Model file for the job. Use its own axes, mm. Face numbers are marked on the shaded views. A direction names the side the tool comes from. Round coordinates to 2 decimals unless told otherwise and drop trailing zeros. Write each loop counter-clockwise with the first axis right and the second up, starting at its lowest first coordinate (ties: lowest second). Pieces come first, ordered by that corner, then holes. Notation, with made-up numbers: (-36.5, -36) - (-23.5, -36) arc R24 ccw to (-23.5, -26) - close; hole circle Ø8 at (11.25, 43.25). An arc over 180 degrees is marked (long way). One line per item, written item: value.
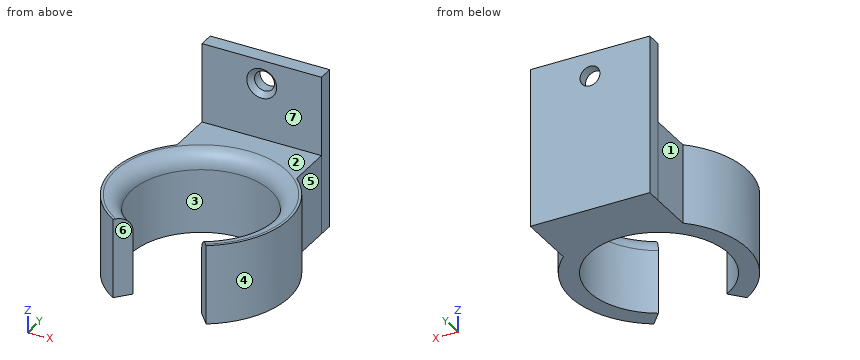
from build123d import *

# Parameters (mm, degrees)
F1_DEPTH       = 25.4
F0_W           = 38.142491
F0_H           = 4.7625
F2_DEPTH       = 50.8
F4_D           = 6.35
F4_CSINK_D     = 9.525
F4_CSINK_ANGLE = 90
F5_R           = 5.08


with BuildPart() as f1:
    # F0 (on Top) → F1 (new body)
    with BuildSketch(Plane.XY):
        with BuildLine():
            Line((-26.27681, 54.485713), (-64.419301, 54.485713))
            Line((-64.419301, 54.485713), (-64.419301, 49.723213))
            Line((-64.419301, 49.723213), (-64.419301, 40.198213))
            ThreePointArc((-64.419301, 40.198213), (-45.348056, 47.647605), (-26.27681, 40.198213))
            Line((-26.27681, 40.198213), (-26.27681, 49.723213))
            Line((-26.27681, 49.723213), (-26.27681, 54.485713))
        make_face()
        with BuildLine():
            ThreePointArc((-26.27681, 40.198213), (-45.348056, 47.647605), (-64.419301, 40.198213))
            ThreePointArc((-64.419301, 40.198213), (-73.361199, 16.87444), (-60.224942, -4.37161))
            Line((-60.224942, -4.37161), (-56.27555, 0.157641))
            ThreePointArc((-56.27555, 0.157641), (-45.348056, 41.73569), (-34.420562, 0.157641))
            Line((-34.420562, 0.157641), (-30.471169, -4.37161))
            ThreePointArc((-30.471169, -4.37161), (-17.334912, 16.87444), (-26.27681, 40.198213))
        make_face()
    extrude(amount=F1_DEPTH)

    # F0 (on Top) → F2 (join)
    with BuildSketch(Plane.XY):
        with Locations((-45.348055, 56.866963)):
            Rectangle(F0_W, F0_H)
    extrude(amount=F2_DEPTH)

    # F4 (through all)
    with Locations(Plane.XZ.offset(-54.485713)):
        with Locations((-45.348056, 43.292329)):
            CounterSinkHole(F4_D / 2, F4_CSINK_D / 2, counter_sink_angle=F4_CSINK_ANGLE)

    # F5
    f5_edges = [f1.edges().sort_by_distance(p)[0] for p in [
        (-45.348056, 41.73569, 25.4),
    ]]
    fillet(f5_edges, radius=F5_R)


solid = f1.part
1. Tool access for the marked faces 4, 5, 6 and 7: list every direction of +Z, -Z, +X, -X, +Y, -Y with a clear straight run to the whole face (end or side of a thin tool).
Report:
face 4: +Z, -Z, +X
face 5: +Z, -Z, +X, +Y
face 6: +Z, -Z, -Y
face 7: +Z, +X, -X, -Y
2. Mould opens along X. For the marked faces 1, 2 and 3 say: released by +X, released by -X, zero draft, split by the parting line, or undercut.
Report:
face 1: released by -X
face 2: zero draft
face 3: undercut
3. Drop flat-ended pins along their axis: pin 1 (15.5 mm diameter, centred on y = 45.5, z = 7.5, fed in from +X); pin 2 (12 mm diameter, centred on x = -38, z = 32.5, fed in from -Y); pin 3 (2 mm diameter, centred on x = -25.5, y = 3.5, fed in from +Z). Give the stop position or say it passes through.
Report:
pin 1: x = -23.92
pin 2: y = 54.49
pin 3: z = 25.34
4. Band-saw the part on B-B on z = 27.5. Write the cut outline in (x, y).
Report:
outline: (-64.42, 54.49) - (-26.28, 54.49) - (-26.28, 59.25) - (-64.42, 59.25) - close
5. Band-saw the part on A-A on z = 19.5. Write the cut outline in (x, y) (3 decimals).
Report:
outline: (-64.419, 40.198) arc R28.137 ccw to (-60.225, -4.372) - (-56.276, 0.158) arc R22.225 cw (long way) to (-34.421, 0.158) - (-30.471, -4.372) arc R28.137 ccw to (-26.277, 40.198) - (-26.277, 59.248) - (-64.419, 59.248) - close
6. Wall check: probe 1 along Y at (x, z) = (-33, 20.5); probe 2 along Y at (x, z) = (-35, 34); probe 3 along X at (y, z) = (55.5, 8.5). Give the ranges that are in metal, low to high. Write a range as [from, to].
Report:
probe 1: [-1.47, 1.03], [37.99, 59.25]
probe 2: [54.49, 59.25]
probe 3: [-64.42, -26.28]
